Could you check a few things on this model? Use its own coordinates, in mm. Face numbers are marked on the shaded views. A direction names the side the tool comes from. Give positions to 0.01 mm unless a question says otherwise; leave off trailing zeros. Order: outer loops, then holes, each group sorted by start corner. A loop starts at its lowest first (then second) coordinate and runs counter-clockwise, first axis right, second up. Notation, with made-up numbers: M 75,78 L 95,78 A22 ccw 95,114 Z; hole C 85.5,22 d6. An arc over 180 degrees is marked long. Use a Markdown table: item, result. Add a question column.
Item 1: If we mould it in two halves opening along Y, with no side actions, what happens to the marked faces 3, 4 and 5? For each: released by +Y, released by -Y, zero draft, split by the parting line, or undercut.
Item 2: If I drill on L1, parallel to Y at x = 6, z = 32.5; L2, parallel to Z at x = 6, y = -24, over which ranges is the centre line in solid material (lowest first)? Write a range as from..to.
Item 3: Suppose I cut it at B-B on x = 8.5. Write out the boundary of the cut face in (y, z).
Item 4: I'm going to push a flat-ended pin straight in: pin 1 Ø1.3 at (x, y) = (-1.5, -39) entering from +Z. Where does the tip first touch, or does it pass through?
Item 5: Suppose I cut it at C-C on y = 24.5. Write out the boundary of the cut face in (x, z).
Item 6: For the marked faces 1 and 2, which set-ups out of +Z, -Z, +X, -X, +Y, -Y let a thin tool reach every point of the face, with its end or its side?
Item 7: Suppose I cut it at A-A on z = 45. Write out the boundary of the cut face in (x, y), plus the area to 3 significant figures.
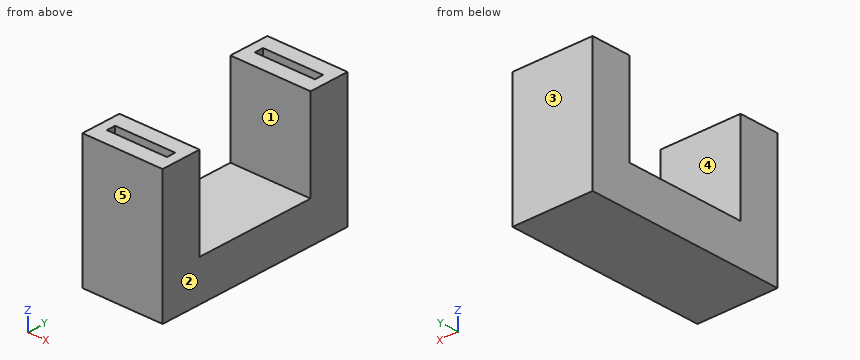
Solid Edge part; units mm, degrees
sketch "Sketch1" plane through (0, 0, 0) normal (0, 0, 1) x (1, 0, 0)
  line L0 (20, -50) -> (20, 50)
  line L1 (20, 50) -> (-20, 50)
  line L2 (-20, 50) -> (-20, -50)
  line L3 (-20, -50) -> (20, -50)
extrude "Protrusion1" add sketch "Sketch1" along normal blind 20
sketch "Sketch2" plane through (0, 0, 20) normal (0, 0, 1) x (1, 0, 0)
  line L0 (-15, 42.25) -> (-15, 37.75)
  line L1 (-15, 37.75) -> (15, 37.75)
  line L2 (15, 37.75) -> (15, 42.25)
  line L3 (15, 42.25) -> (-15, 42.25)
  line L4 (20, 30) -> (-20, 30)
  line L5 (-20, 30) -> (-20, 50)
  line L6 (-20, 50) -> (20, 50)
  line L7 (20, 50) -> (20, 30)
  line L8 (15, -37.75) -> (-15, -37.75)
  line L9 (-15, -37.75) -> (-15, -42.25)
  line L10 (-15, -42.25) -> (15, -42.25)
  line L11 (15, -42.25) -> (15, -37.75)
  line L12 (20, -50) -> (20, -30)
  line L13 (20, -30) -> (-20, -30)
  line L14 (-20, -30) -> (-20, -50)
  line L15 (-20, -50) -> (20, -50)
extrude "Protrusion2" add sketch "Sketch2" along normal blind 45
Findings below:
| question | item | result |
|---|---|---|
| 1 | face 3 | released by +Y |
| 1 | face 4 | undercut |
| 1 | face 5 | released by -Y |
| 2 | L1 | y = -50..-42.25, -37.75..-30, 30..37.75, 42.25..50 |
| 2 | L2 | z = 0..20 |
| 3 | outline | M -50,0 L 50,0 L 50,65 L 42.25,65 L 42.25,20 L 37.75,20 L 37.75,65 L 30,65 L 30,20 L -30,20 L -30,65 L -37.75,65 L -37.75,20 L -42.25,20 L -42.25,65 L -50,65 Z |
| 4 | pin 1 | stops at z = 20 |
| 5 | outline | M -20,0 L 20,0 L 20,20 L -20,20 Z |
| 6 | face 1 | +Z, +X, -X |
| 6 | face 2 | +Z, -Z, +X, +Y, -Y |
| 7 | outline | M -20,-50 L 20,-50 L 20,-30 L -20,-30 Z; M -20,30 L 20,30 L 20,50 L -20,50 Z; hole M -15,-42.25 L 15,-42.25 L 15,-37.75 L -15,-37.75 Z; hole M -15,37.75 L 15,37.75 L 15,42.25 L -15,42.25 Z |
| 7 | area | 1,330 mm^2 |
